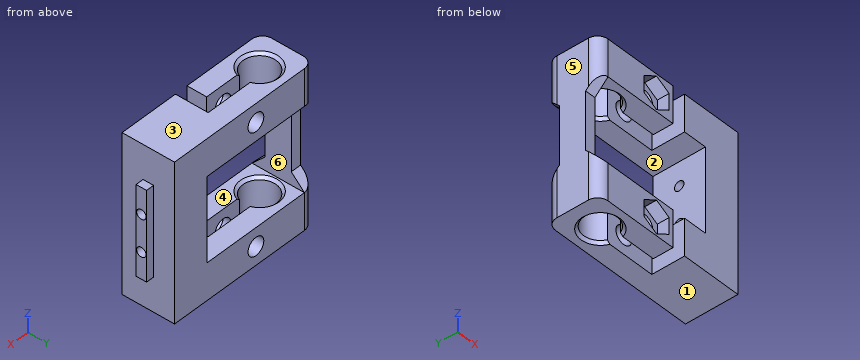
Autodesk Fusion 360 part; units mm, degrees
sketch "Sketch1" plane through (0, 0, 0) normal (0, 1, 0) x (1, 0, 0)
  line L0 (15, 15) -> (-15, 15)
  line L1 (-15, 15) -> (-15, -15)
  line L2 (-15, -15) -> (15, -15)
  line L3 (15, -15) -> (15, 15)
  line L4 (15, 15) -> (-15, -15) construction
  line L5 (-15, 15) -> (15, -15) construction
  dimension "d1" = 30
  dimension "d2" = 30
extrude "Extrude1" add sketch "Sketch1" along normal mid plane 10
sketch "Sketch2" plane through (0, 0, 15) normal (0, 0, 1) x (-1, 0, 0)
  line L0 (-15, 5) -> (-15, -5)
  line L1 (-15, -5) -> (15, -5)
  line L2 (15, -5) -> (15, 5)
  line L3 (15, 5) -> (-15, 5)
  point P0 (9, 0)
  dimension "d5" = 6
hole "Hole1" at (-9, 0, 15) direction (0, 0, -1) diameter 6.35 end through all
sketch "Sketch3" plane through (0, 0, 15) normal (0, 0, 1) x (-1, 0, 0)
  circle A0 centre (9, 0) radius 3.175
  line L0 (-15, 5) -> (-15, -5)
  line L1 (-15, -5) -> (15, -5)
  line L2 (15, -5) -> (15, 5)
  line L3 (15, 5) -> (-15, 5)
  line L4 (-3.5, -1.25) -> (11.5, -1.25)
  line L5 (11.5, -1.25) -> (11.5, 1.25)
  line L6 (11.5, 1.25) -> (-3.5, 1.25)
  line L7 (-3.5, 1.25) -> (-3.5, -1.25)
  line L8 (-3.5, -1.25) -> (11.5, 1.25) construction
  line L9 (11.5, -1.25) -> (-3.5, 1.25) construction
  line L10 (-3.5, 1.25) -> (-1, 1.25)
  line L11 (-1, 1.25) -> (-1, 5)
  line L12 (-3.5, 5) -> (-3.5, 1.25)
  point P0 (4, 0)
  dimension "d9" = 5
  dimension "d10" = 2.5
  dimension "d11" = 15
  dimension "d18" = 2.5
extrude "Extrude2" cut sketch "Sketch3" against normal through all contours A0 L4 L6 L7 L10 | L3 L6 L10 L11 L12
sketch "Sketch4" plane through (0, 5, 0) normal (0, 1, 0) x (-1, 0, 0)
  line L0 (-15, 15) -> (-15, -15)
  line L1 (-15, -15) -> (15, -15)
  line L2 (15, -15) -> (15, 15)
  line L3 (15, 15) -> (-15, 15)
  line L4 (-1, -15) -> (6.0814, -15)
  line L5 (6.0814, -15) -> (6.0814, 15)
  line L6 (6.0814, 15) -> (-1, 15)
  line L7 (-1, 15) -> (-1, -15)
  point P0 (2.5407, 11.5)
  point P1 (2.5407, 15)
  dimension "d14" = 3.5
hole "Hole2" at (-2.5407, 5, 11.5) direction (0, -1, 0) diameter 3.4 depth 10 tip angle 118
sketch "Sketch5" plane through (0, -5, 0) normal (0, -1, 0) x (1, 0, 0)
  circle A0 centre (-2.5407, 11.5) radius 1.7
  line L0 (1, -15) -> (1, 15)
  line L1 (1, 15) -> (-15, 15)
  line L2 (-15, 15) -> (-15, -15)
  line L3 (-15, -15) -> (1, -15)
  line L4 (0.1613, 9.94) -> (0.1613, 13.06)
  line L5 (0.1613, 13.06) -> (-2.5407, 14.62)
  line L6 (-2.5407, 14.62) -> (-5.2427, 13.06)
  line L7 (-5.2427, 13.06) -> (-5.2427, 9.94)
  line L8 (-5.2427, 9.94) -> (-2.5407, 8.38)
  line L9 (-2.5407, 8.38) -> (0.1613, 9.94)
  point P0 (-2.5407, 11.5)
  dimension "d19" = 3.12
extrude "Extrude3" cut sketch "Sketch5" against normal blind 2.25 contours L4 L5 L6 L7 L8 L9
mirror "Mirror1" about plane through (0, 0, 0) normal (0, 0, 1) of "Hole2", "Extrude3"
sketch "Sketch6" plane through (0, 5, 0) normal (0, 1, 0) x (-1, 0, 0)
  circle A0 centre (2.5407, -11.5) radius 1.7
  circle A1 centre (2.5407, 11.5) radius 1.7
  line L0 (-15, 15) -> (-15, -15)
  line L1 (-15, -15) -> (15, -15)
  line L2 (15, -15) -> (15, 15)
  line L3 (15, 15) -> (-15, 15)
  line L4 (13, 8) -> (-8, 8)
  line L5 (-8, 8) -> (-8, -8)
  line L6 (-8, -8) -> (13, -8)
  line L7 (13, -8) -> (13, 8)
  dimension "d24" = 7
  dimension "d25" = 7
  dimension "d26" = 7
  dimension "d27" = 2
extrude "Extrude4" cut sketch "Sketch6" against normal through all contours L4 L5 L6 L7
sketch "Sketch7" plane through (15, 0, 0) normal (1, 0, 0) x (0, 1, 0)
  line L0 (-5, -15) -> (5, -15)
  line L1 (5, -15) -> (5, 15)
  line L2 (5, 15) -> (-5, 15)
  line L3 (-5, 15) -> (-5, -15)
  line L4 (1, -8.5) -> (-1, -8.5)
  line L5 (-1, -8.5) -> (-1, 8.5)
  line L6 (-1, 8.5) -> (1, 8.5)
  line L7 (1, 8.5) -> (1, -8.5)
  line L8 (1, -8.5) -> (-1, 8.5) construction
  line L9 (-1, -8.5) -> (1, 8.5) construction
  dimension "d29" = 2
  dimension "d30" = 17
extrude "Extrude5" add sketch "Sketch7" along normal blind 1.5 contours L4 L5 L6 L7
sketch "Sketch8" plane through (16.5, 0, 0) normal (1, 0, 0) x (0, 1, 0)
  line L0 (1, 8.5) -> (-1, 8.5)
  line L1 (-1, 8.5) -> (-1, -8.5)
  line L2 (-1, -8.5) -> (1, -8.5)
  line L3 (1, -8.5) -> (1, 8.5)
  point P0 (0, 3.5)
  point P1 (0, -3.5)
  dimension "d33" = 3.5
  dimension "d34" = 3.5
hole "Hole3" at (16.5, 0, 3.5) at (16.5, 0, -3.5) direction (-1, 0, 0) diameter 1.8 depth 8.5 tip angle 180
sketch "Sketch9" plane through (-15, 0, 0) normal (-1, 0, 0) x (0, -1, 0)
  line L0 (5, 15) -> (-5, 15)
  line L1 (-5, 15) -> (-5, -15)
  line L2 (-5, -15) -> (5, -15)
  line L3 (5, -15) -> (5, 15)
  line L4 (-5, 8) -> (5, 8)
  line L5 (-5, 8) -> (-2.5, 5.5)
  line L6 (-2.5, 5.5) -> (-2.5, -5.5)
  line L7 (-5, -8) -> (5, -8)
  line L8 (-2.5, -5.5) -> (-5, -8)
  line L9 (-5, 8) -> (-5, -8)
  point P0 (-5, -8)
  dimension "d38" = 135
  dimension "d39" = 135
  dimension "d40" = 2.5
extrude "Extrude6" cut sketch "Sketch9" against normal up to surface (2 mm away) contours L1 L5 L6 L8 L9
chamfer "Chamfer1" distance 0.5 angle 45 4 edges at (-12.175, 0, -15) (-12.175, 0, -8) (-12.175, 0, 8) (-12.175, 0, 15)
mirror "Mirror2" about plane through (0, 0, 0) normal (0, 1, 0) of "Extrude6"
fillet "Fillet1" radius 2 1 edges at (-15, -5, 11.5)
fillet "Fillet1" radius 2 1 edges at (-15, 5, 11.5)
fillet "Fillet1" radius 2 2 edges at (-15, 5, -11.5) (-15, -5, -11.5)
Could you check a few things on this model? Use its own coordinates, in mm. Face numbers are marked on the shaded views. A direction names the side the tool comes from. Round coordinates to 2 decimals unless told otherwise and drop trailing zeros. Write each loop counter-clockwise with the first axis right and the second up, starting at its lowest first coordinate (ties: lowest second). Pieces come first, ordered by that corner, then holes. Notation, with made-up numbers: M 43,-19.5 L 96,-19.5 A9 ccw 96,-12.5 Z; hole C 46,-14 d6. An arc over 180 degrees is marked long. Answer in a Markdown table with one row per item. Add a question column.
Q1. Imagine slicing it at A-A (z = -11.5). Please give me the cut outline in (x, y) (3 decimals).
Q2. If we mould it in two halves opening along Z, with no side actions, what happens to the marked faces 1, 2, 3 and 4? For each: +Z half, -Z half, draft (parallel to the pull), parting line (faces both ways), or undercut.
Q3. If I drill on line 1 (Z direction, x = -12.5, y = -2.25); line 2 (X direction, y = 1.5, z = 5); line 3 (X direction, y = 0, z = -2.5), over which ranges is the centre line in solid material (lowest first)? Write a range as from..to.
Q4. On a 3-axis mill with a long thin cutter (end or side, diameter ignored), from which of +Z, -Z, +X, -X, +Y, -Y can I reach the whole of each face in a straight line? I mean the marked faces 5 and 6. Say none if no direction works.
Q5. Imagine slicing it at D-D (x = -9). Please give me the cut outline in (y, z) (3 decimals).
Q6. Imagine slicing it at B-B (x = 6.5). Please give me the cut outline in (y, z), then the cut area to 3 significant figures.
Q7. Will these pins go through, and if not, where does the flat tip stop? pin 1 Ø1.8 at (y, z) = (-4, -11) entering from +X; pin 2 Ø2 at (x, z) = (-14, -2) entering from -Y; pin 3 Ø4 at (x, y) = (-9, 0) entering from +Z; pin 4 Ø1.4 at (y, z) = (0, 3.5) entering from +X.
Q8. Imagine slicing it at C-C (y = 0). Give the number of separate pieces and of enclosed holes in the cut face, then the cut area to 3 significant figures.
Values:
| question | item | result |
|---|---|---|
| 1 | outline | M -15,-3 A2 ccw -13,-5 L -5.243,-5 L -5.243,-2.75 L -4.241,-2.75 L -4.241,-1.25 L -6.081,-1.25 A3.175 cw long -6.081,1.25 L -4.241,1.25 L -4.241,5 L -13,5 A2 ccw -15,3 Z; M -0.841,-2.75 L 0.161,-2.75 L 0.161,-5 L 1,-5 L 1,-1.25 L -0.841,-1.25 Z; M -0.841,1.25 L 3.5,1.25 L 3.5,-5 L 15,-5 L 15,5 L -0.841,5 Z |
| 2 | face 1 | -Z half |
| 2 | face 2 | undercut |
| 2 | face 3 | +Z half |
| 2 | face 4 | undercut |
| 3 | line 1 | -15..-8, 8..15 |
| 3 | line 2 | -15..-13, 8..15 |
| 3 | line 3 | -15..-13, 8..16.5 |
| 4 | face 5 | +Z, -Z, -X, +Y, -Y |
| 4 | face 6 | +Y, -Y |
| 5 | outline | M -5,-15 L -3.675,-15 L -3.175,-14.5 L -3.175,-8.5 L -3.675,-8 L -5,-8 Z; M -5,8 L -3.675,8 L -3.175,8.5 L -3.175,14.5 L -3.675,15 L -5,15 Z; M 3.175,-14.5 L 3.675,-15 L 5,-15 L 5,-8 L 3.675,-8 L 3.175,-8.5 Z; M 3.175,8.5 L 3.675,8 L 5,8 L 5,15 L 3.675,15 L 3.175,14.5 Z |
| 6 | outline | M -5,-15 L 5,-15 L 5,-8 L -5,-8 Z; M -5,8 L 5,8 L 5,15 L -5,15 Z |
| 6 | area | 140 mm^2 |
| 7 | pin 1 | x = 15 |
| 7 | pin 2 | y = -2.5 |
| 7 | pin 3 | through |
| 7 | pin 4 | x = -13 |
| 8 | separate pieces | 4 |
| 8 | enclosed holes | 0 |
| 8 | area | 339 mm^2 |
